Verification items for this drawing (mm, ordinates from the low corner). A direction names the side the tool comes from. Give positions to 0.01 mm unless a question says otherwise; leave off trailing zeros. Write each loop counter-clockwise with the first axis right and the second up, starting at its lowest first coordinate (ties: lowest second). Pieces come first, ordered by that corner, then holes. Notation, with made-up numbers: (55, -23.75) -> (82, -23.75) arc R16 ccw to (82, -9.75) -> close; hole circle Ø6 at (3.25, 54). An arc over 180 degrees is marked (long way). Use one line per item in the form item = value. Start each with the question number.
(1) Set-up check for the marked faces 5 and 6: record each of +Z, -Z, +X, -X, +Y, -Y from which the full face is reachable in a straight line by a thin tool's end or side.
(2) Scan lines: L1, parallel to Y at x = 31, z = 2.75; L2, parallel to Z at x = 12, y = 21. Record each from-to range of solid material in increasing order.
(3) Depth check by flat-ended pin: pin 1 Ø4 at (y, z) = (19, 5.5) entering from -X. Enter the tip coordinate at first touch or a pass-through.
(4) Section check B-B, the plane z = 8.25. Record the cut outline in (x, y) (1 decimal).
(5) Release check for a two-part mould opening along X. For the marked faces 1, 2, 3 and 4 record: pulls with the +X half, pulls with the -X half, needs draft (parallel to the pull), parting line crosses it, or undercut.
(6) Section check A-A, the plane x = 23.5. Record the cut outline in (y, z), plus the area to 3 significant figures.
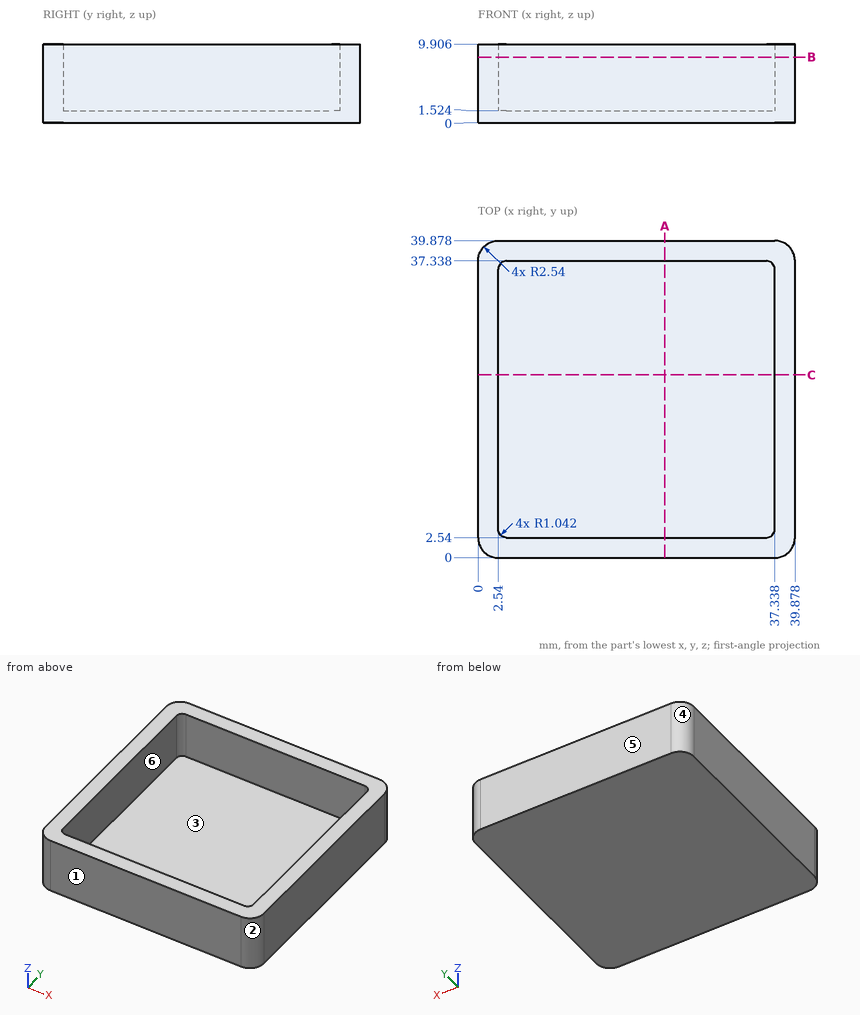
Completed:
q1.face_5 = +Z, -Z, +X, -X, +Y
q1.face_6 = +Z
q2.L1 = 0 to 2.54, 37.34 to 39.88
q2.L2 = 0 to 1.52
q3.pin_1 = 0
q4.outline = (0, 2.5) arc R2.5 ccw to (2.5, 0) -> (37.3, 0) arc R2.5 ccw to (39.9, 2.5) -> (39.9, 37.3) arc R2.5 ccw to (37.3, 39.9) -> (2.5, 39.9) arc R2.5 ccw to (0, 37.3) -> close; hole (2.5, 3.6) arc R1 ccw to (3.6, 2.5) -> (36.3, 2.5) arc R1 ccw to (37.3, 3.6) -> (37.3, 36.3) arc R1 ccw to (36.3, 37.3) -> (3.6, 37.3) arc R1 ccw to (2.5, 36.3) -> close
q5.face_1 = needs draft
q5.face_2 = pulls with the +X half
q5.face_3 = undercut
q5.face_4 = pulls with the -X half
q6.outline = (0, 0) -> (39.88, 0) -> (39.88, 9.91) -> (37.34, 9.91) -> (37.34, 1.52) -> (2.54, 1.52) -> (2.54, 9.91) -> (0, 9.91) -> close
q6.area = 103 mm²
